```python
from build123d import *

# Parameters (mm, degrees)
F0_W     = 16
F0_H     = 4
F1_DEPTH = 57
F3_R     = 2.54
F4_DEPTH = 4.001
F5_R     = 2.54
F6_DEPTH = 84.001


with BuildPart() as f1:
    # F0 (on Top) → F1 (new body)
    with BuildSketch(Plane.XY):
        with Locations((28, 2)):
            Rectangle(F0_W, F0_H)
        Polygon((16, 0), (20, 0), (20, 4), (20, 80), (200, 80), (200, 4), (200, 0), (204, 0), (204, 4), (204, 84), (16, 84), (16, 4), align=None)
        with Locations((192, 2)):
            Rectangle(F0_W, F0_H)
    extrude(amount=F1_DEPTH)

    # F2 (on face) + F3 (on face) → F4 (cut, through all)
    with BuildSketch(Plane(origin=(0, 4, 0), x_dir=(-1, 0, 0), z_dir=(0, 1, 0))):
        with BuildLine():
            ThreePointArc((-23.46, 11.43), (-26, 13.97), (-28.54, 11.43))
            ThreePointArc((-28.54, 11.43), (-26, 8.89), (-23.46, 11.43))
        make_face()
        with BuildLine():
            ThreePointArc((-23.46, 45.57), (-26, 48.11), (-28.54, 45.57))
            ThreePointArc((-28.54, 45.57), (-26, 43.03), (-23.46, 45.57))
        make_face()
    with BuildSketch(Plane(origin=(0, 4, 0), x_dir=(-1, 0, 0), z_dir=(0, 1, 0))):
        with Locations((-194, 11.43)):
            Circle(F3_R)
        with Locations((-194, 45.57)):
            Circle(F3_R)
    extrude(amount=-F4_DEPTH, mode=Mode.SUBTRACT)

    # F5 (on face) → F6 (cut, through all)
    with BuildSketch(Plane(origin=(0, 84, 0), x_dir=(-1, 0, 0), z_dir=(0, 1, 0))):
        with Locations((-173.5, 47.55)):
            Circle(F5_R)
        with Locations((-173.5, 9.45)):
            Circle(F5_R)
        with Locations((-46.5, 9.45)):
            Circle(F5_R)
        with Locations((-46.5, 47.55)):
            Circle(F5_R)
    extrude(amount=-F6_DEPTH, mode=Mode.SUBTRACT)


solid = f1.part
```
The model under review builds one solid part; all positions refer to its coordinate system, in mm. A direction names the side the tool comes from. Round coordinates to 2 decimals unless told otherwise and drop trailing zeros. Order: outer loops, then holes, each group sorted by start corner. A loop starts at its lowest first (then second) coordinate and runs counter-clockwise, first axis right, second up. Notation, with made-up numbers: M -32.5,47.5 L -28.5,47.5 A15 ccw -28.5,51.5 Z; hole C -18,86 d3. An arc over 180 degrees is marked long. Use a Markdown table: item, result.
1) Consider section D-D (z = 30). Write out the cut boundary in (x, y), then the cut area to 3 significant figures.
Report:
| item | result |
|---|---|
| outline | M 16,0 L 36,0 L 36,4 L 20,4 L 20,80 L 200,80 L 200,4 L 184,4 L 184,0 L 204,0 L 204,84 L 16,84 Z |
| area | 1,520 mm^2 |
2) Consider section A-A (y = 14.5). Write out the cut boundary in (x, z), then the cut area to 3 significant figures.
Report:
| item | result |
|---|---|
| outline | M 16,0 L 20,0 L 20,57 L 16,57 Z; M 200,0 L 204,0 L 204,57 L 200,57 Z |
| area | 456 mm^2 |
3) Consider section C-C (x = 194). Write out the cut boundary in (y, z).
Report:
| item | result |
|---|---|
| outline | M 0,0 L 4,0 L 4,8.89 L 0,8.89 Z; M 0,13.97 L 4,13.97 L 4,43.03 L 0,43.03 Z; M 0,48.11 L 4,48.11 L 4,57 L 0,57 Z; M 80,0 L 84,0 L 84,57 L 80,57 Z |
4) Draft analysis for pull direction X (two halves, no side actions). For faces 6 (the face through (28, 4, 28)), 7 (the face through (111, 84, 28)), 8 (the face through (204, 41, 28)), state which applies: released by +X, released by -X, zero draft, split by the parting line, or undercut.
Report:
| item | result |
|---|---|
| face 6 | undercut |
| face 7 | zero draft |
| face 8 | released by +X |
5) Wall thickness on line 1 along Z through (x, y) = (173.5, 82); line 2 along Z through (x, y) = (194, 1); line 3 along X through (y, z) = (54, 26): over which ranges is each line inside the solid? List them lowest first. Write a range as [from, to].
Report:
| item | result |
|---|---|
| line 1 | [0, 6.91], [11.99, 45.01], [50.09, 57] |
| line 2 | [0, 8.89], [13.97, 43.03], [48.11, 57] |
| line 3 | [16, 20], [200, 204] |
6) Tool access review of faces 1 (the face through (36, 2, 28)), 2 (the face through (192.828, 2.028, 43.317)), 3 (the face through (110, 83, 0)), 4 (the face through (20, 41, 28)), 5 (the face through (48.516, 82.028, 46.004)): name each direction out of +Z, -Z, +X, -X, +Y, -Y from which nothing blocks a thin tool from reaching the whole face with its end or side.
Report:
| item | result |
|---|---|
| face 1 | +Z, -Z, -Y |
| face 2 | -Y |
| face 3 | -Z, +X, -X, +Y, -Y |
| face 4 | +Z, -Z |
| face 5 | +Y, -Y |
7) Consider section B-B (x = 173.5). Write out the cut boundary in (y, z), then the cut area to 3 significant figures.
Report:
| item | result |
|---|---|
| outline | M 80,0 L 84,0 L 84,6.91 L 80,6.91 Z; M 80,11.99 L 84,11.99 L 84,45.01 L 80,45.01 Z; M 80,50.09 L 84,50.09 L 84,57 L 80,57 Z |
| area | 187 mm^2 |
8) Insertion check: pin 1 (6.5 mm diameter, centred on x = 194, z = 11.43, fed in from -Y); pin 2 (8 mm diameter, centred on x = 173.5, z = 47.55, fed in from -Y). Each pin has a flat end and moves straight along its axis. Give the tip position at first contact, or say it passes through.
Report:
| item | result |
|---|---|
| pin 1 | y = 0 |
| pin 2 | y = 80 |
